The model under review builds one solid part; all positions refer to its coordinate system, in mm. A direction names the side the tool comes from. Coordinates: 2 decimals unless noted, no trailing zeros. Order: outer loops, then holes, each group sorted by start corner. A loop starts at its lowest first (then second) coordinate and runs counter-clockwise, first axis right, second up.
```python
from build123d import *

# Parameters (mm, degrees)
F0_W     = 41.098144
F0_H     = 45.76838
F2_W     = 8.219628
F2_H     = 32.878513
F3_DEPTH = 22.5
F4_W     = 11.208584
F4_H     = 64.636167
F5_DEPTH = 50
F6_R     = 15.878829
F7_DEPTH = 50


with BuildPart() as f1:
    # F0 (on Top) → F1 (revolve)
    with BuildSketch(Plane.XY):
        with Locations((1.120867, 22.88419)):
            Rectangle(F0_W, F0_H)
    revolve(axis=Axis((1.120867, 0, 0), (1, 0, 0)))

    # F2 (on Right) → F3 (cut, symmetric)
    with BuildSketch(Plane.YZ):
        with Locations((25.966552, -0.747239)):
            Rectangle(F2_W, F2_H)
    extrude(amount=F3_DEPTH, both=True, mode=Mode.SUBTRACT)

    # F4 (on Front) → F5 (cut, symmetric)
    with BuildSketch(Plane.XZ):
        with Locations((0.373617, 0.373619)):
            Rectangle(F4_W, F4_H)
    extrude(amount=F5_DEPTH, both=True, mode=Mode.SUBTRACT)

    # F6 (on Top) → F7 (cut, symmetric)
    with BuildSketch(Plane.XY):
        Circle(F6_R)
    extrude(amount=F7_DEPTH, both=True, mode=Mode.SUBTRACT)


solid = f1.part
```
(1) Machinability: for faces 4 (the face through (-12, 26, 15.692)), 5 (the face through (5.978, 33, 0)), which of the approach directions +Z, -Z, +X, -X, +Y, -Y give a long, thin tool a straight path to every point of the face, cutting with its end or side? Answer none if there is none.
A:
face 4: +X, -X
face 5: +Y, -Y
(2) For pin 1 Ø9 at (x, y) = (3, 22.5) entering from -Z; pin 2 Ø9 at (x, y) = (-10, 27.5) entering from +Z; pin 3 Ø4.5 at (x, z) = (16.5, -4) entering from -Y, all flat-tipped, find the tip position at first contact; note any pin that passes through.
A:
pin 1: stops at z = -42.08
pin 2: stops at z = 39.57
pin 3: stops at y = -45.73
(3) We need section A-A, the plane x = -7.5. Write out the cut boundary in (y, z).
A:
outline: (-14, -43.58) - (-14, 43.58) arc R45.77 ccw to start; (14, -43.58) arc R45.77 ccw to (14, 43.58) - close; hole (21.86, -17.19) - (30.08, -17.19) - (30.08, 15.69) - (21.86, 15.69) - close
(4) We need section B-B, the plane y = 0. Write out the cut boundary in (x, z).
A:
outline: (-19.43, -45.77) - (-15.88, -45.77) - (-15.88, 45.77) - (-19.43, 45.77) - close; (15.88, -45.77) - (21.67, -45.77) - (21.67, 45.77) - (15.88, 45.77) - close
(5) Draft analysis for pull direction Y (two halves, no side actions). For faces 1 (the face through (14.67, -6.08, 0.64)), 2 (the face through (21.67, 1, 1)), 3 (the face through (10.541, 43.655, 13.748)), state which applies: released by +Y, released by -Y, zero draft, split by the parting line, or undercut.
A:
face 1: undercut
face 2: zero draft
face 3: split by the parting line
(6) We need section C-C, the plane z = 0. Write out the cut boundary in (x, y), and give its area (3 significant figures).
A:
outline: (-19.43, -45.77) - (-5.23, -45.77) - (-5.23, -14.99) arc R15.88 cw to (-5.23, 14.99) - (-5.23, 21.86) - (-19.43, 21.86) - close; (-19.43, 30.08) - (-5.23, 30.08) - (-5.23, 45.77) - (-19.43, 45.77) - close; (5.98, -45.77) - (21.67, -45.77) - (21.67, 21.86) - (5.98, 21.86) - (5.98, 14.71) arc R15.88 cw to (5.98, -14.71) - close; (5.98, 30.08) - (21.67, 30.08) - (21.67, 45.77) - (5.98, 45.77) - close
area: 2,050 mm2
(7) We need section D-D, the plane x = -2. Write out the cut boundary in (y, z).
A:
outline: (-32.78, -31.94) arc R45.77 ccw to (-15.75, -42.97) - (-15.75, -31.94) - close; (-32.03, 32.69) - (-15.75, 32.69) - (-15.75, 42.97) arc R45.77 ccw to start; (15.75, -42.97) arc R45.77 ccw to (32.78, -31.94) - (15.75, -31.94) - close; (15.75, 32.69) - (32.03, 32.69) arc R45.77 ccw to (15.75, 42.97) - close
(8) Wall thickness on probe 1 along X at (y, z) = (0, -6); probe 2 along Y at (x, z) = (14, 11.5); probe 3 along Y at (x, z) = (13, 12): over which ranges is each line inside the solid? List them lowest first.
A:
probe 1: x = -19.43 to -15.88, 15.88 to 21.67
probe 2: y = -44.3 to -7.49, 7.49 to 21.86, 30.08 to 44.3
probe 3: y = -44.17 to -9.12, 9.12 to 21.86, 30.08 to 44.17
